Check sheet for the drawn part. Datum: minimum x, y, z corner. Units: mm. Round coordinates to 2 decimals unless told otherwise and drop trailing zeros. Write each loop counter-clockwise with the first axis right and the second up, starting at its lowest first coordinate (ties: lowest second). Pieces come first, ordered by that corner, then holes. Notation, with made-up numbers: (-21.5, 59.25) - (7.5, 59.25) arc R28 ccw to (7.5, 98.25) - close; hole circle Ø9 at (-16.5, 62.25). An arc over 180 degrees is marked (long way). Answer as a JSON object with one key per item and string values.
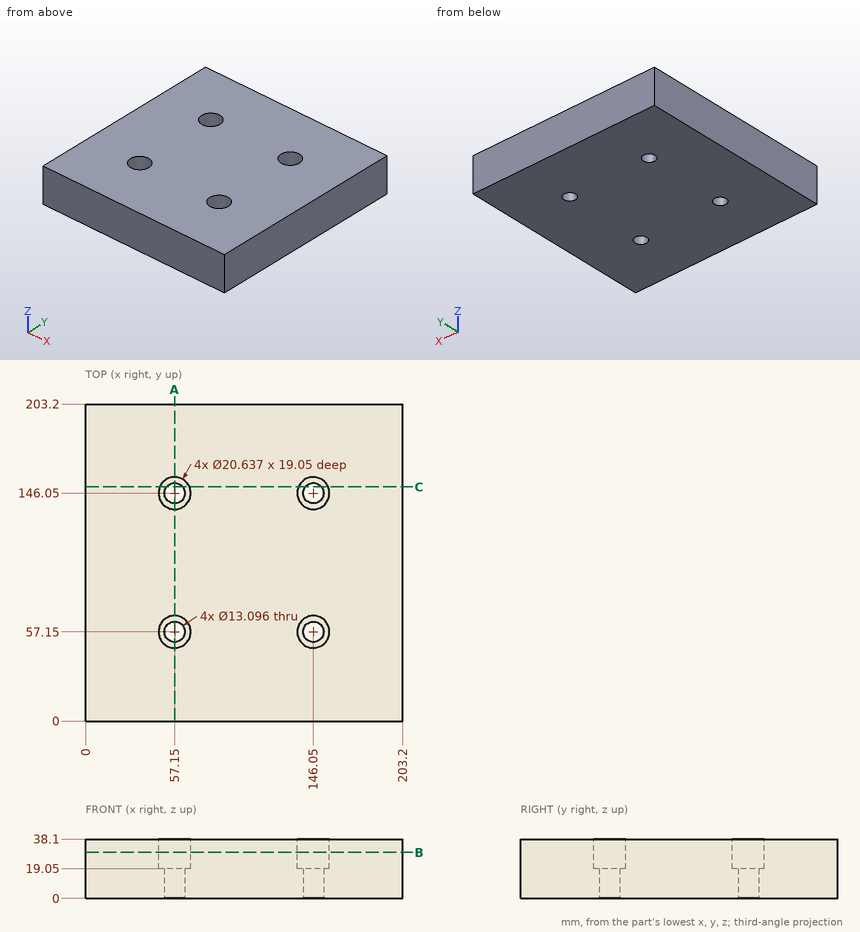
Q1. Gauge pin test, flat ends, axial feed: P1, Ø1.5, axis at y = 135.5, z = 30, coming from the -X side; P2, Ø17, axis at x = 57.15, y = 57.15, coming from the +Z side. Record the tip position at first contact, or that the pin passes through.
Geometry check:
{"P1": "stops at x = 0", "P2": "stops at z = 19.05"}
Q2. Section check C-C, the plane y = 150. Record the cut outline in (x, z).
Geometry check:
{"outline": "(0, 0) - (51.93, 0) - (51.93, 19.05) - (47.62, 19.05) - (47.62, 38.1) - (0, 38.1) - close; (62.37, 0) - (140.83, 0) - (140.83, 19.05) - (136.52, 19.05) - (136.52, 38.1) - (66.68, 38.1) - (66.68, 19.05) - (62.37, 19.05) - close; (151.27, 0) - (203.2, 0) - (203.2, 38.1) - (155.58, 38.1) - (155.58, 19.05) - (151.27, 19.05) - close"}
Q3. Section check B-B, the plane z = 29.5. Record the cut outline in (x, y).
Geometry check:
{"outline": "(0, 0) - (203.2, 0) - (203.2, 203.2) - (0, 203.2) - close; hole circle Ø20.64 at (57.15, 57.15); hole circle Ø20.64 at (57.15, 146.05); hole circle Ø20.64 at (146.05, 57.15); hole circle Ø20.64 at (146.05, 146.05)"}
Q4. Material ranges on line 1 along Y through (x, z) = (57.15, 25); line 2 along X through (y, z) = (146.5, 25); line 3 along X through (y, z) = (146.05, 7.5), recorded low to high. Write a range as [from, to].
Geometry check:
{"line 1": "y = [0, 46.83], [67.47, 135.73], [156.37, 203.2]", "line 2": "x = [0, 46.84], [67.46, 135.74], [156.36, 203.2]", "line 3": "x = [0, 50.6], [63.7, 139.5], [152.6, 203.2]"}
Q5. Section check A-A, the plane x = 57.15. Record the cut outline in (y, z), then the cut area to 3 significant figures.
Geometry check:
{"outline": "(0, 0) - (50.6, 0) - (50.6, 19.05) - (46.83, 19.05) - (46.83, 38.1) - (0, 38.1) - close; (63.7, 0) - (139.5, 0) - (139.5, 19.05) - (135.73, 19.05) - (135.73, 38.1) - (67.47, 38.1) - (67.47, 19.05) - (63.7, 19.05) - close; (152.6, 0) - (203.2, 0) - (203.2, 38.1) - (156.37, 38.1) - (156.37, 19.05) - (152.6, 19.05) - close", "area": "6,460 mm2"}
